Model file for the job. Use its own axes, mm. Face numbers are marked on the shaded views. Give positions to 0.01 mm unless a question says otherwise; leave off trailing zeros. Loops run counter-clockwise (first coordinate to the right, second up) from the corner with the lowest first, then second, coordinate; pieces in that order, holes last. Notation, with made-up numbers: M 35.5,10.5 L 93.5,10.5 A8 cw 93.5,21.5 Z; hole C 80,54 d4. An arc over 180 degrees is marked long. Answer in a Markdown table with one row per item.
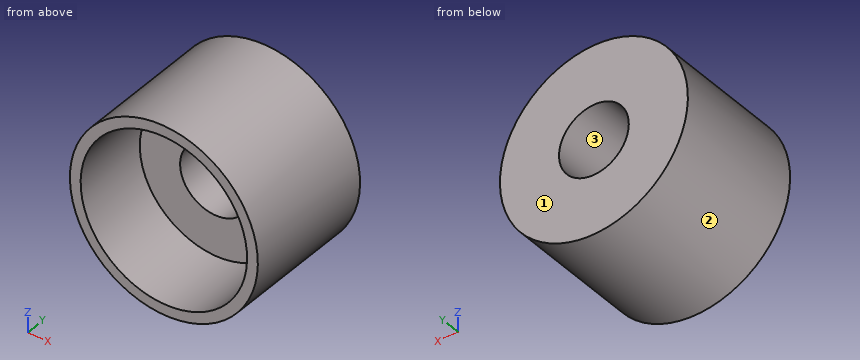
```python
from build123d import *

# Parameters (mm, degrees)
SKETCH018_R         = 35
PAD013_DEPTH        = 50
SKETCH019_R         = 31
POCKET002_DEPTH     = 45
SKETCH020_R         = 28
PAD014_DEPTH        = 20
SKETCH021_R         = 13
POCKET003_DEPTH     = 25.001
BODY010_ROLL_ANGLE  = -90
BODY010_PITCH_ANGLE = -5


with BuildPart() as part:
    # Sketch018 → Pad013 (new body)
    with BuildSketch(Plane.XY):
        Circle(SKETCH018_R)
    extrude(amount=PAD013_DEPTH)

    # Sketch019 (on Face2 of Pad013) → Pocket002 (cut)
    with BuildSketch(Plane(origin=(0, 0, 0), x_dir=(1, 0, 0), z_dir=(0, 0, -1))):
        Circle(SKETCH019_R)
    extrude(amount=-POCKET002_DEPTH, mode=Mode.SUBTRACT)

    # Sketch020 (on Face5 of Pocket002) → Pad014 (join)
    with BuildSketch(Plane(origin=(0, 0, 45), x_dir=(1, 0, 0), z_dir=(0, 0, -1))):
        Circle(SKETCH020_R)
    extrude(amount=PAD014_DEPTH)

    # Sketch021 (on Face7 of Pad014) → Pocket003 (cut, through all)
    with BuildSketch(Plane(origin=(0, 0, 25), x_dir=(1, 0, 0), z_dir=(0, 0, -1))):
        Circle(SKETCH021_R)
    extrude(amount=-POCKET003_DEPTH, mode=Mode.SUBTRACT)


with BuildPart() as part_1:
    # Body010 roll: moved
    add(part.part.rotate(Axis((0, 0, 0), (1, 0, 0)), BODY010_ROLL_ANGLE))


with BuildPart() as part_2:
    # Body010 pitch: moved
    add(part_1.part.rotate(Axis((0, 0, 0), (0, 1, 0)), BODY010_PITCH_ANGLE))


with BuildPart() as part_3:
    # Body010 placement: moved
    add(part_2.part.moved(Location((0, -199.6, 0))))


solid = part_3.part
```
(1) Mould opens along X. For the marked faces 1, 2 and 3 say: pulls with the +X half, pulls with the -X half, needs draft (parallel to the pull), parting line crosses it, or undercut.
Established:
| item | result |
|---|---|
| face 1 | needs draft |
| face 2 | parting line crosses it |
| face 3 | undercut |
(2) Saw through at B-B, the plane z = 0. Give the cut face in (x, y).
Established:
| item | result |
|---|---|
| outline | M -35,-199.6 L -31,-199.6 L -31,-154.6 L -28,-154.6 L -28,-174.6 L -13,-174.6 L -13,-149.6 L -35,-149.6 Z; M 13,-174.6 L 28,-174.6 L 28,-154.6 L 31,-154.6 L 31,-199.6 L 35,-199.6 L 35,-149.6 L 13,-149.6 Z |
(3) Saw through at D-D, the plane z = 20. Give the cut face in (x, y).
Established:
| item | result |
|---|---|
| outline | M -28.72,-199.6 L -23.69,-199.6 L -23.69,-154.6 L -19.6,-154.6 L -19.6,-174.6 L 19.6,-174.6 L 19.6,-154.6 L 23.69,-154.6 L 23.69,-199.6 L 28.72,-199.6 L 28.72,-149.6 L -28.72,-149.6 Z |
(4) Wall check: L1, parallel to X at y = -168.5, z = 0; L2, parallel to Z at x = 0, y = -177; L3, parallel to X at y = -158, z = -2.5. Give the ranges that are in metal, low to high.
Established:
| item | result |
|---|---|
| L1 | x = -35 to -31, -28 to -13, 13 to 28, 31 to 35 |
| L2 | z = -35 to -31, 31 to 35 |
| L3 | x = -34.91 to -30.9, -27.89 to -12.76, 12.76 to 27.89, 30.9 to 34.91 |
(5) Saw through at A-A, the plane x = 0. Give the cut face in (y, z).
Established:
| item | result |
|---|---|
| outline | M -199.6,-35 L -149.6,-35 L -149.6,-13 L -174.6,-13 L -174.6,-28 L -154.6,-28 L -154.6,-31 L -199.6,-31 Z; M -199.6,31 L -154.6,31 L -154.6,28 L -174.6,28 L -174.6,13 L -149.6,13 L -149.6,35 L -199.6,35 Z |
(6) Flat gauge pins, fed straight in: P1, Ø1.5, axis at y = -180.5, z = -13.5, coming from the -X side; P2, Ø2, axis at y = -176, z = 24.5, coming from the +X side; P3, Ø5, axis at x = 19, y = -184.5, coming from the -Z side. Where does each tip first touch, or does it go through?
Established:
| item | result |
|---|---|
| P1 | stops at x = -32.6 |
| P2 | stops at x = 25.94 |
| P3 | stops at z = -30.87 |
(7) Saw through at C-C, the plane x = 23.5. Give the cut face in (y, z).
Established:
| item | result |
|---|---|
| outline | M -199.6,-25.94 L -149.6,-25.94 L -149.6,25.94 L -199.6,25.94 L -199.6,20.22 L -154.6,20.22 L -154.6,15.22 L -174.6,15.22 L -174.6,-15.22 L -154.6,-15.22 L -154.6,-20.22 L -199.6,-20.22 Z |
